```python
from build123d import *

# Parameters (mm, degrees)
BOSS_EXTRUDE1_DEPTH      = 3.5
BOSS_EXTRUDE1_DEPTH_BACK = 3.5
SKETCH1_R                = 16.05
BOSS_EXTRUDE2_START      = 0.8
SKETCH2_R                = 14
BOSS_EXTRUDE2_DEPTH      = 0.8
SKETCH3_R                = 1.4
CUT_EXTRUDE1_DEPTH       = 55.80823387
FILLET1_R                = 2


with BuildPart() as part:
    # Sketch1 → Boss-Extrude1 (new, two sides: drawn at the far end of the back side and taken through both)
    with BuildSketch(Plane.XY.offset(-BOSS_EXTRUDE1_DEPTH_BACK)):
        with BuildLine():
            Line((0, 21.05), (-50, 21.05))
            Line((-50, 21.05), (-50, -21.05))
            Line((-50, -21.05), (0, -21.05))
            ThreePointArc((0, -21.05), (21.05, 0), (0, 21.05))
        make_face()
        Circle(SKETCH1_R, mode=Mode.SUBTRACT)
    extrude(amount=BOSS_EXTRUDE1_DEPTH + BOSS_EXTRUDE1_DEPTH_BACK)

    # Sketch2 → Boss-Extrude2 (add)
    with BuildSketch(Plane(origin=(0, 0, -3.5), x_dir=(-1, 0, 0), z_dir=(0, 0, -1)).offset(BOSS_EXTRUDE2_START)):
        with BuildLine():
            Line((0, -21.05), (50, -21.05))
            Line((50, -21.05), (50, 21.05))
            Line((50, 21.05), (0, 21.05))
            ThreePointArc((0, 21.05), (-21.05, 0), (0, -21.05))
        make_face()
        Circle(SKETCH2_R, mode=Mode.SUBTRACT)
    extrude(amount=-BOSS_EXTRUDE2_DEPTH)

    # Sketch3 → Cut-Extrude1 (cut, through all)
    with BuildSketch(Plane(origin=(0, 0, -4.3), x_dir=(-1, 0, 0), z_dir=(0, 0, -1))):
        with Locations((20, 16.05)):
            Circle(SKETCH3_R)
        with Locations((45, 16.05)):
            Circle(SKETCH3_R)
        with Locations((45, -16.05)):
            Circle(SKETCH3_R)
        with Locations((20, -16.05)):
            Circle(SKETCH3_R)
    extrude(amount=-CUT_EXTRUDE1_DEPTH, mode=Mode.SUBTRACT)

    # Fillet1
    fillet1_edges = [part.edges().sort_by_distance(p)[0] for p in [
        (-50, -21.05, -0.4),
        (-50, 21.05, -0.4),
    ]]
    fillet(fillet1_edges, radius=FILLET1_R)


solid = part.part
```
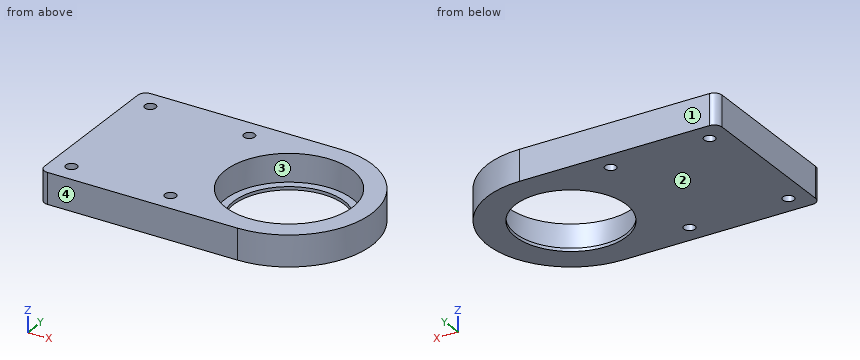
Input: part model. Units: mm. Frame: model coordinates. Face numbers are marked on the shaded views. Coordinates: 2 decimals unless noted, no trailing zeros. Loops run counter-clockwise (first coordinate to the right, second up) from the corner with the lowest first, then second, coordinate; pieces in that order, holes last.
Q1. Line query: line 1 along Y through (x, z) = (-45, -0.5); line 2 along X through (y, z) = (0.5, -0.5); line 3 along X through (y, z) = (-17, 3). Output: solid intervals per line, ascending.
Results are:
line 1: y = -21.05 to -17.45, -14.65 to 14.65, 17.45 to 21.05
line 2: x = -50 to -16.04, 16.04 to 21.04
line 3: x = -50 to -46.03, -43.97 to -21.03, -18.97 to 12.41
Q2. Section C-C, the plane x = -20. Return the cut outline in (y, z).
Results are:
outline: (-21.05, -4.3) - (-17.45, -4.3) - (-17.45, 3.5) - (-21.05, 3.5) - close; (-14.65, -4.3) - (14.65, -4.3) - (14.65, 3.5) - (-14.65, 3.5) - close; (17.45, -4.3) - (21.05, -4.3) - (21.05, 3.5) - (17.45, 3.5) - close
Q3. Contact query for flat-ended pins moving along their axis: pin 1 (16 mm diameter, centred on x = -6.5, y = 4.5, fed in from +Z); pin 2 (10 mm diameter, centred on x = 9, y = 1, fed in from -Z); pin 3 (2 mm diameter, centred on y = 3.5, z = -3.5, fed in from +X); pin 4 (1 mm diameter, centred on y = -15.5, z = 2.5, fed in from +X). Output: stop coordinate, or through.
Results are:
pin 1: stops at z = -3.5
pin 2: stops at z = -4.3
pin 3: stops at x = 20.9
pin 4: stops at x = 14.77
Q4. Section A-A, the plane z = 0.25. Return the cut outline in (x, y).
Results are:
outline: (-50, -19.05) arc R2 ccw to (-48, -21.05) - (0, -21.05) arc R21.05 ccw to (0, 21.05) - (-48, 21.05) arc R2 ccw to (-50, 19.05) - close; hole circle Ø2.8 at (-45, -16.05); hole circle Ø2.8 at (-45, 16.05); hole circle Ø2.8 at (-20, -16.05); hole circle Ø2.8 at (-20, 16.05); hole circle Ø32.1 at (0, 0)
Q5. Mould query, pull axis Y, two halves, no side actions, for the marked faces 1, 2, 3 and 4. Classes: +Y half, -Y half, draft (parallel to the pull), parting line (faces both ways), or undercut.
Results are:
face 1: +Y half
face 2: draft
face 3: undercut
face 4: -Y half
Q6. Section D-D, the plane x = -8. Return the cut outline in (y, z).
Results are:
outline: (-21.05, -4.3) - (-11.49, -4.3) - (-11.49, -3.5) - (-13.91, -3.5) - (-13.91, 3.5) - (-21.05, 3.5) - close; (11.49, -4.3) - (21.05, -4.3) - (21.05, 3.5) - (13.91, 3.5) - (13.91, -3.5) - (11.49, -3.5) - close
Q7. Section B-B, the plane y = 0. Return the cut outline in (x, z), and give its area (3 significant figures).
Results are:
outline: (-50, -4.3) - (-14, -4.3) - (-14, -3.5) - (-16.05, -3.5) - (-16.05, 3.5) - (-50, 3.5) - close; (14, -4.3) - (21.05, -4.3) - (21.05, 3.5) - (16.05, 3.5) - (16.05, -3.5) - (14, -3.5) - close
area: 307 mm2
